Input: part model. Units: mm. Frame: model coordinates. A direction names the side the tool comes from. Round coordinates to 2 decimals unless told otherwise and drop trailing zeros. Loops run counter-clockwise (first coordinate to the right, second up) from the corner with the lowest first, then second, coordinate; pieces in that order, holes last. Notation, with made-up numbers: M 47.25,61.25 L 92.25,61.25 A25 ccw 92.25,85.25 Z; hole C 69.25,-14.5 d10. An arc over 180 degrees is marked long. Use one line per item in the form item = value. Start each with the question number.
Q1. Access query for faces 5 (the cylindrical face through (160.88, 14.71, 18.73)), 6 (the flat face through (98.6, -3.5, 3)), 7 (the flat face through (8, 37, 20)). Directions: +Z, -Z, +X, -X, +Y, -Y. A direction counts if a zero-diameter tool reaches every point of the face in a straight line with its end or side. Return the directions, or none.
Q2. First-contact query: P1, Ø12, axis at x = 153.5, z = 22, coming from the +Y side; P2, Ø6, axis at y = 7.5, z = 29.5, coming from the -X side; P3, Ø12.5, axis at x = 10, z = 23.5, coming from the -Y side. Flat tips, straight axial feed; report the tip coordinate or a pass-through.
Q3. Ray query, line 1 along Y through (x, z) = (15, 2.25); line 2 along Z through (x, y) = (86, -15); line 3 along X through (y, z) = (21.5, 8). Return the intervals inside material, ascending.
Q4. Mould query, pull axis X, two halves, no side actions, for faces 1 (the flat face through (100, 0, 19)), 2 (the flat face through (100, -3, 20)), 3 (the cylindrical face through (161.076, 11.102, 20.255)), 4 (the cylindrical face through (39.88, 14.13, 18.73)). Classes: pulls with the +X half, pulls with the -X half, needs draft (parallel to the pull), parting line crosses it, or undercut.
Q5. Section query C-C, the plane z = 24. Output: boundary loops of the cut face in (x, y).
Q6. Section query A-A, the plane y = 12.5. Output: boundary loops of the cut face in (x, z).
Q7. Section query D-D, the plane y = -6. Output: boundary loops of the cut face in (x, z), and give its area (3 significant figures).
Q8. Section query B-B, the plane x = 105.5. Output: boundary loops of the cut face in (y, z), and give its area (3 significant figures).
```python
from build123d import *

# Parameters (mm, degrees)
SKETCH_1_W          = 200
SKETCH_1_H          = 30
EXTRUDE_1_DEPTH     = 3
SKETCH_2_R          = 1.5
CUT_EXTRUDE_1_DEPTH = 3
EXTRUDE_2_DEPTH     = 35


with BuildPart() as part:
    # 草图1 → 凸台-拉伸1 (new body)
    with BuildSketch(Plane.XY):
        with Locations((100, -15)):
            Rectangle(SKETCH_1_W, SKETCH_1_H)
        with BuildLine():
            Line((0, 40), (0, 0))
            Line((0, 0), (70, 0))
            ThreePointArc((70, 0), (39.497390629, 14.4184502), (17.5, 40))
            Line((17.5, 40), (0, 40))
        make_face()
        with BuildLine():
            ThreePointArc((182.5, 40), (160.502609371, 14.4184502), (130, 0))
            Line((130, 0), (200, 0))
            Line((200, 0), (200, 40))
            Line((200, 40), (182.5, 40))
        make_face()
    extrude(amount=EXTRUDE_1_DEPTH)

    # 草图2 → 切除-拉伸1 (cut)
    with BuildSketch(Plane.XY.offset(3)):
        with Locations((185, -20)):
            Circle(SKETCH_2_R)
        with Locations((100, -20)):
            Circle(SKETCH_2_R)
        with Locations((15, -20)):
            Circle(SKETCH_2_R)
    extrude(amount=-CUT_EXTRUDE_1_DEPTH, mode=Mode.SUBTRACT)

    # 草图15 → 凸台-拉伸2 (add)
    with BuildSketch(Plane.XY.offset(3)):
        with BuildLine():
            Line((69.653562136, -3), (130.346437864, -3))
            ThreePointArc((130.346437864, -3), (161.46492885, 11.388677272), (184.25647691, 37))
            Line((184.25647691, 37), (200, 37))
            Line((200, 37), (200, 40))
            Line((200, 40), (182.5, 40))
            ThreePointArc((182.5, 40), (160.502609371, 14.4184502), (130, 0))
            Line((130, 0), (70, 0))
            ThreePointArc((70, 0), (39.497390629, 14.4184502), (17.5, 40))
            Line((17.5, 40), (0, 40))
            Line((0, 40), (0, 37))
            Line((0, 37), (15.74352309, 37))
            ThreePointArc((15.74352309, 37), (38.53507115, 11.388677272), (69.653562136, -3))
        make_face()
    extrude(amount=EXTRUDE_2_DEPTH)


solid = part.part
```
Results found:
q1.face_5 = +Z, -Z, +Y
q1.face_6 = +Z, -Y
q1.face_7 = +Z, -X, -Y
q2.P1 = 13.67
q2.P2 = 39.76
q2.P3 = 36.13
q3.line_1 = -30 to -21.5, -18.5 to 40
q3.line_2 = 0 to 3
q3.line_3 = 27.21 to 31.38, 168.62 to 172.79
q4.face_1 = undercut
q4.face_2 = needs draft
q4.face_3 = pulls with the +X half
q4.face_4 = undercut
q5.outline = M 0,37 L 15.74,37 A84.11 ccw 69.65,-3 L 130.35,-3 A84.11 ccw 184.26,37 L 200,37 L 200,40 L 182.5,40 A81.11 cw 130,0 L 70,0 A81.11 cw 17.5,40 L 0,40 Z
q6.outline = M 0,0 L 42.12,0 L 42.12,38 L 37.07,38 L 37.07,3 L 0,3 Z; M 157.88,0 L 200,0 L 200,3 L 162.93,3 L 162.93,38 L 157.88,38 Z
q7.outline = M 0,0 L 200,0 L 200,3 L 0,3 Z
q7.area = 600 mm²
q8.outline = M -30,0 L 0,0 L 0,38 L -3,38 L -3,3 L -30,3 Z
q8.area = 195 mm²
